Design review of the part shown in the three views and the two pictorial views. Dimensions are in mm from the part's minimum x, y and z. A direction names the side the tool comes from. Give positions to 0.01 mm unless a question says otherwise; leave off trailing zeros. Order: outer loops, then holes, each group sorted by start corner. A loop starts at its lowest first (then second) coordinate and runs counter-clockwise, first axis right, second up.
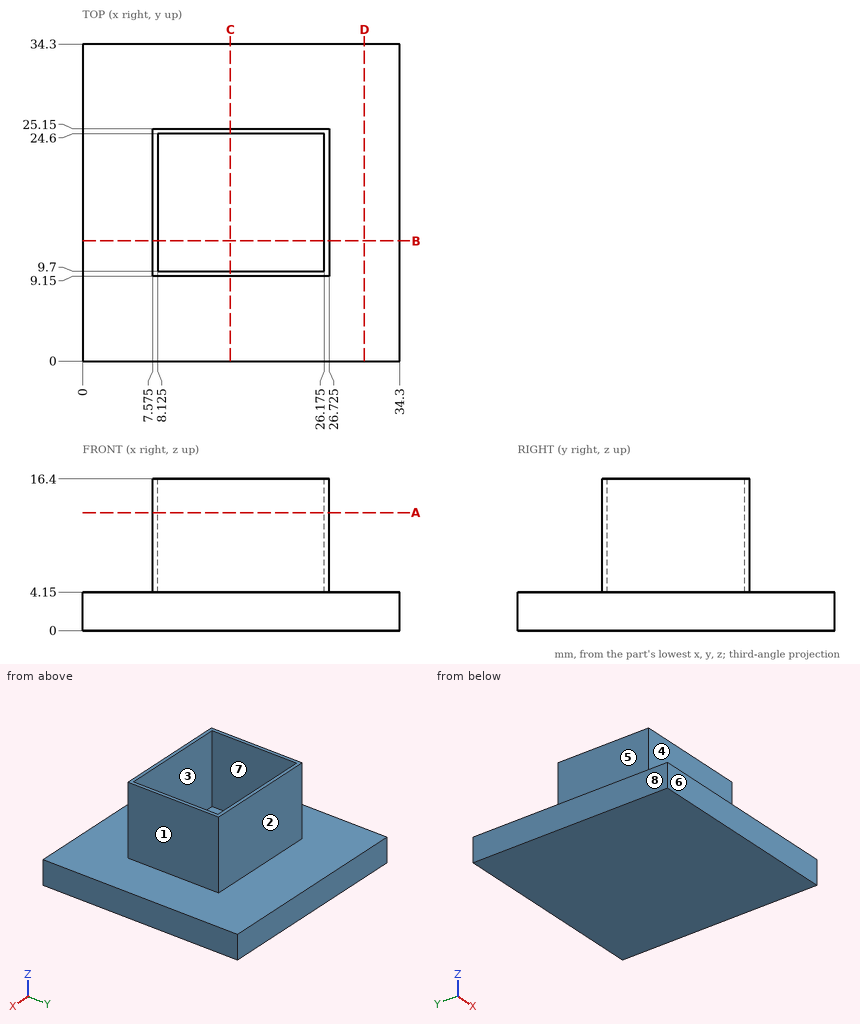
1) Clearance check with flat-ended pins moving along their axes: pin 1 (2 mm diameter, centred on y = 21, z = 7.5, fed in from +X) (3 decimals); pin 2 (3.5 mm diameter, centred on x = 16, z = 10.5, fed in from +Y); pin 3 (5 mm diameter, centred on y = 12.5, z = 12, fed in from -X) (3 decimals); pin 4 (1 mm diameter, centred on x = 28.5, z = 5, fed in from +Y). State where each tip first meets the part, or that it passes through.
Answer sheet:
pin 1: stops at x = 26.725
pin 2: stops at y = 25.15
pin 3: stops at x = 7.575
pin 4: passes through
2) We need section A-A on z = 12.75. Give the boundary of the cut face in (x, y) (3 decimals).
Answer sheet:
outline: (7.575, 9.15) - (26.725, 9.15) - (26.725, 25.15) - (7.575, 25.15) - close; hole (8.125, 9.7) - (26.175, 9.7) - (26.175, 24.6) - (8.125, 24.6) - close
3) We need section C-C on x = 16. Give the boundary of the cut face in (y, z), then the cut area to 3 significant figures.
Answer sheet:
outline: (0, 0) - (34.3, 0) - (34.3, 4.15) - (25.15, 4.15) - (25.15, 16.4) - (24.6, 16.4) - (24.6, 4.15) - (9.7, 4.15) - (9.7, 16.4) - (9.15, 16.4) - (9.15, 4.15) - (0, 4.15) - close
area: 156 mm2
4) Draft analysis for pull direction X (two halves, no side actions). For the marked faces 6, 7 and 8, state which applies: +X half, -X half, draft (parallel to the pull), parting line (faces both ways), or undercut.
Answer sheet:
face 6: draft
face 7: undercut
face 8: -X half
5) To check wall thickness, follow line 1 (Y direction, x = 24, z = 8); line 2 (X direction, y = 19.5, z = 12) (3 decimals); line 3 (Z direction, x = 11.5, y = 12). State the ranges of each line that lie inside material, in increasing order.
Answer sheet:
line 1: y = 9.15 to 9.7, 24.6 to 25.15
line 2: x = 7.575 to 8.125, 26.175 to 26.725
line 3: z = 0 to 4.15
6) We need section D-D on x = 30.5. Give the boundary of the cut face in (y, z), then the cut area to 3 significant figures.
Answer sheet:
outline: (0, 0) - (34.3, 0) - (34.3, 4.15) - (0, 4.15) - close
area: 142 mm2
7) We need section B-B on y = 13. Give the boundary of the cut face in (x, z) (3 decimals), then the cut area to 3 significant figures.
Answer sheet:
outline: (0, 0) - (34.3, 0) - (34.3, 4.15) - (26.725, 4.15) - (26.725, 16.4) - (26.175, 16.4) - (26.175, 4.15) - (8.125, 4.15) - (8.125, 16.4) - (7.575, 16.4) - (7.575, 4.15) - (0, 4.15) - close
area: 156 mm2
8) Tool access review of the marked faces 1, 2, 3, 4 and 5: name each direction out of +Z, -Z, +X, -X, +Y, -Y from which nothing blocks a thin tool from reaching the whole face with its end or side.
Answer sheet:
face 1: +Z, +X, +Y, -Y
face 2: +Z, +X, -X, +Y
face 3: +Z
face 4: +Z, +X, -X, -Y
face 5: +Z, -X, +Y, -Y
